from build123d import *

# Parameters (mm, degrees)
EXTRUSION1_DEPTH = 20
HOLE2_D          = 6.8


with BuildPart() as part:
    # Sketch1 → Extrusion1 (new body)
    with BuildSketch(Plane.XY):
        Polygon((2.963546137, 0.389938146), (-0.346853863, 3.700338146), (-0.346853863, 6.545138146), (3.652646137, 6.545138146), (3.652646137, 9.389938146), (11.653646137, 9.389938146), (11.653646137, 6.545138146), (15.653146137, 6.545138146), (15.653146137, 3.700338146), (12.342746137, 0.389938146), align=None)
    extrude(amount=EXTRUSION1_DEPTH)

    # Hole2 (through all)
    with Locations(Plane.XZ.offset(-0.389938146)):
        with Locations((7.653146137, 10)):
            Hole(HOLE2_D / 2)


solid = part.part
Source: CAD feature listing. Evaluate the final solid. Frame: model axes, mm. A direction names the side the tool comes from. Round coordinates to 2 decimals unless told otherwise and drop trailing zeros. Write each loop counter-clockwise with the first axis right and the second up, starting at its lowest first coordinate (ties: lowest second). Pieces come first, ordered by that corner, then holes. Notation, with made-up numbers: (66.25, 70) - (70.25, 70) arc R22 cw to (70.25, 87) - close; hole circle Ø10 at (7, -24). An arc over 180 degrees is marked (long way). Use CSV: the item, a comma, the result in double quotes. Start each with the question number.
(1) Material intervals for probe 1 along Z at (x, y) = (5.25, 8.75); probe 2 along Z at (x, y) = (8.75, 1.5); probe 3 along X at (y, z) = (7.75, 18.25), sorted ascending. Write a range as [from, to].
(2) Set-up query: faces 4 (the face through (14.02, 2.07, 9.86)), 5 (the face through (11.654, 8, 10)), 6 (the face through (2, 6.545, 10)). Return all of +Z, -Z, +X, -X, +Y, -Y with unobstructed straight access to the full face (end or side cutting, diameter ignored); none if empty.
(3) First-contact query: pin 1 Ø1.2 at (x, z) = (1, 11.5) entering from +Y; pin 2 Ø0.9 at (y, z) = (8, 13.5) entering from +X. Flat tips, straight axial feed; report the tip coordinate or a pass-through.
(4) Mould query, pull axis Z, two halves, no side actions, for faces 1 (the face through (8.39, 4.95, 6.68)), 2 (the face through (8, 5, 0)), 3 (the face through (14, 6.545, 10)). Classes: pulls with the +Z half, pulls with the -Z half, needs draft (parallel to the pull), parting line crosses it, or undercut.
(5) Cut plane A-A, the plane z = 10. Return loops of the section in (x, y), and give its area (3 significant figures).
(6) Cut plane C-C, the plane z = 2. Return loops of the section in (x, y), and give its area (3 significant figures).
(7) Cut plane D-D, the plane y = 8.75. Return loops of the section in (x, z).
(8) Cut plane B-B, the plane x = 7.25. Return loops of the section in (y, z), and give its area (3 significant figures).
Geometry says:
1,probe 1,"[0, 7.59], [12.41, 20]"
1,probe 2,"[0, 6.78], [13.22, 20]"
1,probe 3,"[3.65, 11.65]"
2,face 4,"+Z, -Z, +X, -Y"
2,face 5,"+Z, -Z, +X, +Y"
2,face 6,"+Z, -Z, -X, +Y"
3,pin 1,"y = 6.55"
3,pin 2,"x = 11.65"
4,face 1,"undercut"
4,face 2,"pulls with the -Z half"
4,face 3,"needs draft"
5,outline,"(-0.35, 3.7) - (2.96, 0.39) - (4.25, 0.39) - (4.25, 9.39) - (3.65, 9.39) - (3.65, 6.55) - (-0.35, 6.55) - close; (11.05, 0.39) - (12.34, 0.39) - (15.65, 3.7) - (15.65, 6.55) - (11.65, 6.55) - (11.65, 9.39) - (11.05, 9.39) - close"
5,area,"49.1 mm²"
6,outline,"(-0.35, 3.7) - (2.96, 0.39) - (12.34, 0.39) - (15.65, 3.7) - (15.65, 6.55) - (11.65, 6.55) - (11.65, 9.39) - (3.65, 9.39) - (3.65, 6.55) - (-0.35, 6.55) - close"
6,area,"110 mm²"
7,outline,"(3.65, 0) - (11.65, 0) - (11.65, 20) - (3.65, 20) - close; hole circle Ø6.8 at (7.65, 10)"
8,outline,"(0.39, 0) - (9.39, 0) - (9.39, 6.62) - (0.39, 6.62) - close; (0.39, 13.38) - (9.39, 13.38) - (9.39, 20) - (0.39, 20) - close"
8,area,"119 mm²"
